```python
from build123d import *

# Parameters (mm, degrees)
SKETCH1_R                                           = 35
SKETCH1_R_2                                         = 10
BOSS_EXTRUDE1_DEPTH                                 = 30
SKETCH4_R                                           = 12.5
CUT_EXTRUDE2_DEPTH                                  = 15
CBORE_FOR_M6_HEX_SOCKET_HEAD_CAP_SCREW1_D           = 6.4
CBORE_FOR_M6_HEX_SOCKET_HEAD_CAP_SCREW1_CBORE_D     = 11
CBORE_FOR_M6_HEX_SOCKET_HEAD_CAP_SCREW1_CBORE_DEPTH = 8.4
F_8_0MM_DOWEL_HOLE1_D                               = 8
SKETCH14_OUTSIDE_W                                  = 92.688
SKETCH14_OUTSIDE_H                                  = 92.688
SKETCH14_OUTSIDE_W_2                                = 70
SKETCH14_OUTSIDE_H_2                                = 25.4
CUT_EXTRUDE3_DEPTH                                  = 2
SKETCH18_R                                          = 2.1
CUT_EXTRUDE5_DEPTH                                  = 3
CUT_EXTRUDE6_DEPTH                                  = 58.879184825
CUT_EXTRUDE6_DEPTH_BACK                             = 58.879184825
BOSS_EXTRUDE2_DEPTH                                 = 2
DRAFT1_ANGLE                                        = 15
FILLET1_R                                           = 10


with BuildPart() as part:
    # Sketch1 → Boss-Extrude1 (new body)
    with BuildSketch(Plane(origin=(0, 0, 0), x_dir=(1, 0, 0), z_dir=(0, 1, 0))):
        with Locations(Location((0, 0, 0), (0, 0, 270))):
            Circle(SKETCH1_R)
        with Locations(Location((0, 0, 0), (0, 0, 270))):
            Circle(SKETCH1_R_2, mode=Mode.SUBTRACT)
    extrude(amount=-BOSS_EXTRUDE1_DEPTH)

    # Sketch4 → Cut-Extrude2 (cut)
    with BuildSketch(Plane(origin=(0, 0, 0), x_dir=(1, 0, 0), z_dir=(0, 1, 0))):
        with Locations(Location((0, 0, 0), (0, 0, 270))):
            Circle(SKETCH4_R)
    extrude(amount=-CUT_EXTRUDE2_DEPTH, mode=Mode.SUBTRACT)

    # CBORE for M6 Hex Socket Head Cap Screw1 (through all)
    with Locations(Plane(origin=(0, -30, 0), x_dir=(-1, 0, 0), z_dir=(0, -1, 0))):
        with Locations((0, 25), (21.650635095, -12.5), (-21.650635095, -12.5)):
            CounterBoreHole(CBORE_FOR_M6_HEX_SOCKET_HEAD_CAP_SCREW1_D / 2, CBORE_FOR_M6_HEX_SOCKET_HEAD_CAP_SCREW1_CBORE_D / 2, CBORE_FOR_M6_HEX_SOCKET_HEAD_CAP_SCREW1_CBORE_DEPTH)

    # Ø8.0mm Dowel Hole1 (through all)
    with Locations(Plane(origin=(0, -30, 0), x_dir=(-1, 0, 0), z_dir=(0, -1, 0))):
        with Locations((13.75, -23.815698604), (-13.75, 23.815698604)):
            Hole(F_8_0MM_DOWEL_HOLE1_D / 2)

    # Sketch14 outside → Cut-Extrude3 (cut)
    with BuildSketch(Plane.XZ.offset(30)):
        Rectangle(SKETCH14_OUTSIDE_W, SKETCH14_OUTSIDE_H)
        Rectangle(SKETCH14_OUTSIDE_W_2, SKETCH14_OUTSIDE_H_2, mode=Mode.SUBTRACT)
    extrude(amount=-CUT_EXTRUDE3_DEPTH, mode=Mode.SUBTRACT)

    # Sketch18 → Cut-Extrude5 (cut)
    with BuildSketch(Plane.XZ.offset(30)):
        with Locations(Location((-13.665, 0, 0), (0, 0, 270))):
            Circle(SKETCH18_R)
    extrude(amount=-CUT_EXTRUDE5_DEPTH, mode=Mode.SUBTRACT)

    # Sketch19 → Cut-Extrude6 (cut, two sides: drawn at the far end of the back side and taken through both)
    with BuildSketch(Plane(origin=(0, 0, 0), x_dir=(0, 0, -1), z_dir=(1, 0, 0)).offset(-CUT_EXTRUDE6_DEPTH_BACK)):
        Polygon((-12.7, -28), (-12.164101615, -30), (-12.7, -30), align=None)
        Polygon((12.7, -28), (12.164101615, -30), (12.7, -30), align=None)
    extrude(amount=CUT_EXTRUDE6_DEPTH + CUT_EXTRUDE6_DEPTH_BACK, mode=Mode.SUBTRACT)

    # Sketch20 → Boss-Extrude2 (add)
    with BuildSketch(Plane.XZ.offset(30)):
        with BuildLine():
            Line((-12.581122044, 12.164101615), (12.581122044, 12.164101615))
            ThreePointArc((12.581122044, 12.164101615), (0, 17.5), (-12.581122044, 12.164101615))
        make_face()
        with BuildLine():
            Line((-12.581122044, -12.164101615), (12.581122044, -12.164101615))
            ThreePointArc((12.581122044, -12.164101615), (0, -17.5), (-12.581122044, -12.164101615))
        make_face()
    extrude(amount=-BOSS_EXTRUDE2_DEPTH)

    # Draft1
    draft1_faces = [part.faces().sort_by_distance(p)[0] for p in [
        (0, -29, 17.5),
        (0, -29, -17.5),
    ]]
    draft(draft1_faces, Plane(origin=(0, -28, 0), x_dir=(0, 0, -1), z_dir=(0, -1, 0)), DRAFT1_ANGLE)

    # Fillet1
    fillet1_edges = [part.edges().sort_by_distance(p)[0] for p in [
        (11.932625996, -29.000048438, 12.432037829),
        (-11.932625996, -29.000048438, 12.432037829),
        (-11.932625996, -29.000048438, -12.432037829),
        (11.932625996, -29.000048438, -12.432037829),
    ]]
    fillet(fillet1_edges, radius=FILLET1_R)


solid = part.part
```
The model under review builds one solid part; all positions refer to its coordinate system, in mm. A direction names the side the tool comes from. Coordinates: 2 decimals unless noted, no trailing zeros. Write each loop counter-clockwise with the first axis right and the second up, starting at its lowest first coordinate (ties: lowest second). Pieces come first, ordered by that corner, then holes.
1) We need section B-B on x = 0. State the section outline as (y, z) points.
2) We need section C-C on y = -9. State the section outline as (x, z) points, then the cut area to 3 significant figures.
3) To check wall thickness, follow probe 1 along X at (y, z) = (-4.25, 0); probe 2 along X at (y, z) = (-20.5, -23.5); probe 3 along X at (y, z) = (-22, 0). State the ranges of each line that lie inside material, in increasing order.
4) We need section D-D on x = -22.5. State the section outline as (y, z) points, then the cut area to 3 significant figures.
5) The part is to be moulded in two halves that separate along Z. For faces 5 (the face through (-24.156, -28.986, -12.436)), 6 (the face through (-11.583, -28.521, 0.273)), 7 (the face through (0, -28, 24)), say which applies: pulls with the +Z half, pulls with the -Z half, needs draft (parallel to the pull), parting line crosses it, or undercut.
6) We need section A-A on z = 0. State the section outline as (x, y) points (3 decimals).
7) Machinability: for faces 1 (the face through (23.91, -28.986, -12.436)), 2 (the face through (0, -28, -19)), 3 (the face through (-2.4, -21.6, -22.6)), 4 (the face through (10.2, -15, -0.1)), which of the approach directions +Z, -Z, +X, -X, +Y, -Y give a long, thin tool a straight path to every point of the face, cutting with its end or side? Answer none if there is none.
8) Clearance check with flat-ended pins moving along their axes: pin 1 Ø12 at (y, z) = (-21, 13) entering from +X; pin 2 Ø10 at (x, z) = (21.65, 12.5) entering from +Y; pin 3 Ø2 at (x, y) = (-3, -24.5) entering from +Z; pin 4 Ø3.5 at (x, z) = (-22, 11) entering from -Y. State where each tip first meets the part, or that it passes through.
Answer list:
1. outline: (-30, -16.96) - (-28, -17.5) - (-28, -19.5) - (-21.6, -19.5) - (-21.6, -21.8) - (0, -21.8) - (0, -12.5) - (-15, -12.5) - (-15, -10) - (-30, -10) - close; (-30, 10) - (-15, 10) - (-15, 12.5) - (0, 12.5) - (0, 35) - (-28, 35) - (-28, 17.5) - (-30, 16.96) - close; (-28, -35) - (0, -35) - (0, -28.2) - (-21.6, -28.2) - (-21.6, -30.5) - (-28, -30.5) - close
2. outline: circle Ø70 at (0, 0); hole circle Ø6.4 at (-21.65, 12.5); hole circle Ø8 at (-13.75, 23.82); hole circle Ø25 at (0, 0); hole circle Ø6.4 at (0, -25); hole circle Ø8 at (13.75, -23.82); hole circle Ø6.4 at (21.65, 12.5)
2. area: 3,160 mm2
3. probe 1: x = -35 to -12.5, 12.5 to 35
3. probe 2: x = -25.94 to -2.83, 2.83 to 9.76, 17.74 to 25.94
3. probe 3: x = -35 to -10, 10 to 35
4. outline: (-30, -12.16) - (-28, -12.7) - (-28, -26.81) - (0, -26.81) - (0, 9.41) - (-21.6, 9.41) - (-21.6, 7.07) - (-30, 7.07) - close; (-28, 17.93) - (-21.6, 17.93) - (-21.6, 15.59) - (0, 15.59) - (0, 26.81) - (-28, 26.81) - close
4. area: 1,340 mm2
5. face 5: pulls with the -Z half
5. face 6: undercut
5. face 7: needs draft
6. outline: (-35, -30) - (-15.765, -30) - (-15.765, -27) - (-11.565, -27) - (-11.565, -30) - (-10, -30) - (-10, -15) - (-12.5, -15) - (-12.5, 0) - (-35, 0) - close; (10, -30) - (35, -30) - (35, 0) - (12.5, 0) - (12.5, -15) - (10, -15) - close
7. face 1: -Z, +X, -Y
7. face 2: -Z, -Y
7. face 3: -Y
7. face 4: +Y
8. pin 1: stops at x = 34.29
8. pin 2: stops at y = 0
8. pin 3: stops at z = 34.94
8. pin 4: stops at y = -21.6
